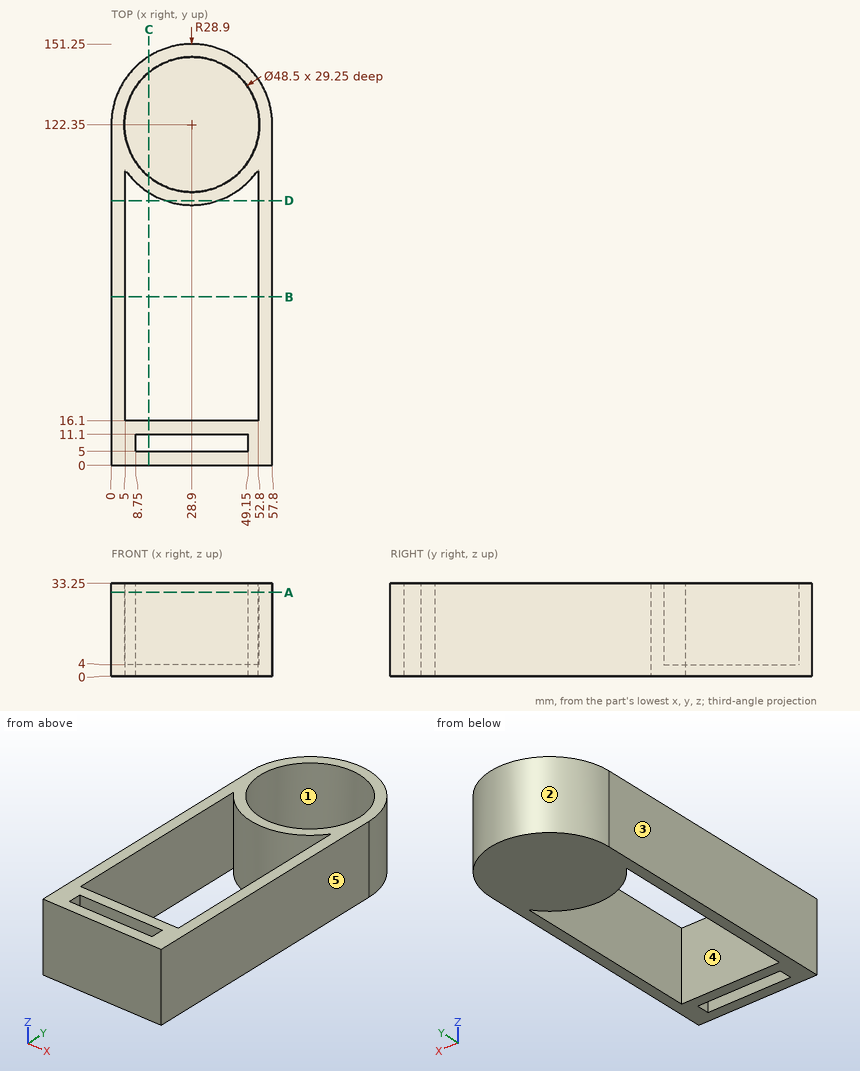
Geometry: see drawing. Coordinates: mm, zero at the bounding-box minimum. A direction names the side the tool comes from. Coordinates: 2 decimals unless noted, no trailing zeros. Order: outer loops, then holes, each group sorted by start corner. A loop starts at its lowest first (then second) coordinate and runs counter-clockwise, first axis right, second up. Notation, with made-up numbers: M 22.25,37 L 76.25,37 A31 cw 76.25,67 Z; hole C -34,19.25 d4. An arc over 180 degrees is marked long. Answer in a Markdown table with one row per item. Add a question column.
Q1. Mould query, pull axis Y, two halves, no side actions, for the marked faces 1, 2 and 3. Classes: released by +Y, released by -Y, zero draft, split by the parting line, or undercut.
Q2. Section query C-C on x = 13.5. Return the cut outline in (y, z), and give its area (3 significant figures).
Q3. Line query: L1, parallel to Y at x = 28, z = 26; L2, parallel to X at y = 122, z = 25; L3, parallel to X at y = 65.5, z = 13. Output: solid intervals per line, ascending.
Q4. Section query B-B on y = 60.5. Return the cut outline in (x, z).
Q5. Section query D-D on y = 95. Return the cut outline in (x, z).
Q6. Section query A-A on z = 30. Return the cut outline in (x, y).
Q7. Contact query for flat-ended pins moving along their axis: P1, Ø16.5, axis at x = 19.5, z = 11, coming from the +Y side; P2, Ø6, axis at x = 43, y = 122, coming from the +Z side. Output: stop coordinate, or through.
Q8. Reachability of the marked faces 4 and 5 from +Z, -Z, +X, -X, +Y, -Y: full face, straight path, thin tool, end or side. Return the list, or none.
Completed:
| question | item | result |
|---|---|---|
| 1 | face 1 | undercut |
| 1 | face 2 | released by +Y |
| 1 | face 3 | zero draft |
| 2 | outline | M 0,0 L 5,0 L 5,33.25 L 0,33.25 Z; M 11.1,0 L 16.1,0 L 16.1,33.25 L 11.1,33.25 Z; M 97.89,0 L 146.81,0 L 146.81,33.25 L 141.08,33.25 L 141.08,4 L 103.62,4 L 103.62,33.25 L 97.89,33.25 Z |
| 2 | area | 863 mm2 |
| 3 | L1 | y = 0 to 5, 11.1 to 16.1, 93.46 to 98.12, 146.58 to 151.24 |
| 3 | L2 | x = 0 to 4.65, 53.15 to 57.8 |
| 3 | L3 | x = 0 to 5, 52.8 to 57.8 |
| 4 | outline | M 0,0 L 5,0 L 5,33.25 L 0,33.25 Z; M 52.8,0 L 57.8,0 L 57.8,33.25 L 52.8,33.25 Z |
| 5 | outline | M 0,0 L 5,0 L 5,33.25 L 0,33.25 Z; M 19.56,0 L 38.24,0 L 38.24,33.25 L 19.56,33.25 Z; M 52.8,0 L 57.8,0 L 57.8,33.25 L 52.8,33.25 Z |
| 6 | outline | M 0,0 L 57.8,0 L 57.8,122.35 A28.9 ccw 0,122.35 Z; hole C 28.9,122.35 d48.5; hole M 5,16.1 L 52.8,16.1 L 52.8,106.1 A28.9 cw 5,106.1 Z; hole M 8.75,5 L 49.15,5 L 49.15,11.1 L 8.75,11.1 Z |
| 7 | P1 | stops at y = 151.23 |
| 7 | P2 | stops at z = 4 |
| 8 | face 4 | +Z, -Z |
| 8 | face 5 | +Z, -Z, +X, +Y, -Y |
